```python
from build123d import *

# Parameters (mm, degrees)
F1_DEPTH = 114.3
F2_W     = 472.44
F2_H     = 104.14
F3_DEPTH = 374.904
F4_W     = 114.3
F4_H     = 63.5
F5_DEPTH = 25.4


with BuildPart() as f1:
    # F0 (on Front) → F1 (new body)
    with BuildSketch(Plane.XZ):
        Polygon((-241.3, -190.5), (241.3, -190.5), (241.3, 190.5), (57.15, 190.5), (57.15, 0), (-57.15, 0), (-57.15, 190.5), (-241.3, 190.5), align=None)
    extrude(amount=-F1_DEPTH)

    # F2 (on face) → F3 (cut)
    with BuildSketch(Plane.XY.offset(190.5)):
        with Locations((0, 57.15)):
            Rectangle(F2_W, F2_H)
    extrude(amount=-F3_DEPTH, mode=Mode.SUBTRACT)

    # F4 (on face) → F5 (cut)
    with BuildSketch(Plane.XZ):
        with Locations((0, -31.75)):
            Rectangle(F4_W, F4_H)
    extrude(amount=-F5_DEPTH, mode=Mode.SUBTRACT)


solid = f1.part
```
Geometry check sheet. Reference: the model listing, model coordinates, mm. A direction names the side the tool comes from. Coordinates: 2 decimals unless noted, no trailing zeros. Write each loop counter-clockwise with the first axis right and the second up, starting at its lowest first coordinate (ties: lowest second). Pieces come first, ordered by that corner, then holes. Notation, with made-up numbers: M 83.5,-6.75 L 113.5,-6.75 A25 ccw 113.5,22.25 Z; hole C -25,44.5 d7. An arc over 180 degrees is marked long. One line per item, written item: value. Start each with the question number.
(1) Tool access check on faces 1 (the face through (241.3, 56, -3)), 2 (the face through (-3, 5.08, -78)). Record the directions out of +Z, -Z, +X, -X, +Y, -Y that give a thin tool (end or side, any length) a straight path to the whole face; none if there is none.
(2) Sectioned sample at B-B, the plane y = 17. Enter the section's corners in (x, z), and give its area (3 significant figures).
(3) Release check for a two-part mould opening along X. For faces 3 (the face through (-3, 56, -190.5)), 4 (the face through (-241.3, 56, 3)), 5 (the face through (-3, 58, -184.404)) record: released by +X, released by -X, zero draft, split by the parting line, or undercut.
(4) Sectioned sample at A-A, the plane z = 36.5. Enter the section's corners in (x, y), and give its area (3 significant figures).
(5) Scan lines: line 1 along Y through (x, z) = (-135, 68); line 2 along X through (y, z) = (46, 170.5); line 3 along Z through (x, y) = (179.5, 39). Record each from-to range of solid material in increasing order. Write a range as [from, to].
(6) Depth check by flat-ended pin: pin 1 (12 mm diameter, centred on x = 118, z = 151, fed in from -Y); pin 2 (2.5 mm diameter, centred on x = 28.5, y = 3, fed in from +Z); pin 3 (5.5 mm diameter, centred on x = -11.5, y = 112, fed in from +Z). Enter the tip coordinate at first touch or a pass-through.
(7) Sectioned sample at C-C, the plane z = -96.5. Enter the section's corners in (x, y), and give its area (3 significant figures).
(8) Sectioned sample at D-D, the plane x = 102. Enter the section's corners in (y, z).
Filled sheet:
1. face 1: +Z, -Z, +X, +Y, -Y
1. face 2: +Z
2. outline: M -241.3,-190.5 L 241.3,-190.5 L 241.3,190.5 L 236.22,190.5 L 236.22,-184.4 L -236.22,-184.4 L -236.22,190.5 L -241.3,190.5 Z
2. area: 6,750 mm²
3. face 3: zero draft
3. face 4: released by -X
3. face 5: undercut
4. outline: M -241.3,0 L -57.15,0 L -57.15,5.08 L -236.22,5.08 L -236.22,109.22 L -57.15,109.22 L -57.15,114.3 L -241.3,114.3 Z; M 57.15,0 L 241.3,0 L 241.3,114.3 L 57.15,114.3 L 57.15,109.22 L 236.22,109.22 L 236.22,5.08 L 57.15,5.08 Z
4. area: 4,800 mm²
5. line 1: [0, 5.08], [109.22, 114.3]
5. line 2: [-241.3, -236.22], [236.22, 241.3]
5. line 3: [-190.5, -184.4]
6. pin 1: y = 0
6. pin 2: z = -63.5
6. pin 3: z = 0
7. outline: M -241.3,0 L 241.3,0 L 241.3,114.3 L -241.3,114.3 Z; hole M -236.22,5.08 L 236.22,5.08 L 236.22,109.22 L -236.22,109.22 Z
7. area: 5,960 mm²
8. outline: M 0,-190.5 L 114.3,-190.5 L 114.3,190.5 L 109.22,190.5 L 109.22,-184.4 L 5.08,-184.4 L 5.08,190.5 L 0,190.5 Z
